Part model, mm, in its own coordinate system. A direction names the side the tool comes from. Round coordinates to 2 decimals unless told otherwise and drop trailing zeros. Loops run counter-clockwise (first coordinate to the right, second up) from the corner with the lowest first, then second, coordinate; pieces in that order, holes last.
from build123d import *

# Parameters (mm, degrees)
SKETCH1_R           = 1.7
BOSS_EXTRUDE1_DEPTH = 70
SKETCH2_W           = 60
SKETCH2_H           = 10
CUT_EXTRUDE1_DEPTH  = 25
BOSS_EXTRUDE2_DEPTH = 5
SKETCH4_W           = 10
SKETCH4_H           = 60
CUT_EXTRUDE2_DEPTH  = 20
BOSS_EXTRUDE3_DEPTH = 5


with BuildPart() as part:
    # Sketch1 → Boss-Extrude1 (new body)
    with BuildSketch(Plane.XY.offset(246.476360497)):
        Polygon((-42.55341426, 305.4352577), (-42.55341426, 275.4352577), (-22.55341426, 275.4352577), (-22.55341426, 285.4352577), (-12.649269186, 285.4352577), (-12.649269186, 305.4352577), align=None)
        with Locations((-17.55341426, 295.4352577)):
            Circle(SKETCH1_R, mode=Mode.SUBTRACT)
        with Locations((-32.55341426, 280.4352577)):
            Circle(SKETCH1_R, mode=Mode.SUBTRACT)
    extrude(amount=BOSS_EXTRUDE1_DEPTH)

    # Sketch2 → Cut-Extrude1 (cut)
    with BuildSketch(Plane.ZY.offset(42.55341426)):
        with Locations((281.476360497, 280.4352577)):
            Rectangle(SKETCH2_W, SKETCH2_H)
    extrude(amount=-CUT_EXTRUDE1_DEPTH, mode=Mode.SUBTRACT)

    # Sketch3 → Boss-Extrude2 (add)
    with BuildSketch(Plane.ZY.offset(42.55341426)):
        Polygon((311.476360497, 275.4352577), (301.476360497, 285.4352577), (261.476360497, 285.4352577), (251.476360497, 275.4352577), (246.476360497, 275.4352577), (246.476360497, 305.4352577), (316.476360497, 305.4352577), (316.476360497, 275.4352577), align=None)
    extrude(amount=-BOSS_EXTRUDE2_DEPTH)

    # Sketch4 → Cut-Extrude2 (cut)
    with BuildSketch(Plane(origin=(0, 305.4352577, 0), x_dir=(1, 0, 0), z_dir=(0, 1, 0))):
        with Locations((-17.649269186, -281.476360497)):
            Rectangle(SKETCH4_W, SKETCH4_H)
    extrude(amount=-CUT_EXTRUDE2_DEPTH, mode=Mode.SUBTRACT)

    # Sketch5 → Boss-Extrude3 (add)
    with BuildSketch(Plane(origin=(0, 305.4352577, 0), x_dir=(1, 0, 0), z_dir=(0, 1, 0))):
        Polygon((-12.649269186, -311.476360497), (-22.649269186, -301.476360497), (-22.649269186, -261.476360497), (-12.649269186, -251.476360497), (-12.649269186, -246.476360497), (-42.55341426, -246.476360497), (-42.55341426, -316.476360497), (-12.649269186, -316.476360497), align=None)
    extrude(amount=-BOSS_EXTRUDE3_DEPTH)


solid = part.part
1) Slice it at B-B, the plane x = -24.5. Give the cut face in (y, z).
Values:
outline: (275.44, 246.48) - (305.44, 246.48) - (305.44, 316.48) - (275.44, 316.48) - (275.44, 311.48) - (285.44, 311.48) - (285.44, 251.48) - (275.44, 251.48) - close
2) Wall check: line 1 along Z through (x, y) = (-15.25, 294.75); line 2 along Y through (x, z) = (-16, 254); line 3 along X through (y, z) = (289, 294). Give the ranges that are in metal, low to high.
Values:
line 1: z = 246.48 to 251.48, 311.48 to 316.48
line 2: y = 300.44 to 305.44
line 3: x = -42.55 to -22.65
3) Drop flat-ended pins along their axis: pin 1 Ø2.5 at (x, z) = (-15.5, 313.5) entering from -Y; pin 2 Ø16 at (y, z) = (296.5, 292) entering from +X; pin 3 Ø3 at (x, y) = (-32.55, 280.44) entering from +Z; pin 4 Ø8 at (y, z) = (279, 256) entering from +X. Give the stop position or say it passes through.
Values:
pin 1: stops at y = 285.44
pin 2: stops at x = -22.65
pin 3: passes through
pin 4: stops at x = -37.55
4) Tool access for faces 1 (the face through (-20, 300.435, 309)), 2 (the face through (-17.579, 302.97, 306.546)), 3 (the face through (-22.553, 280, 249)), 4 (the face through (-40.088, 280.365, 306.546)): list every direction of +Z, -Z, +X, -X, +Y, -Y with a clear straight run to the whole face (end or side of a thin tool).
Values:
face 1: +X, -Y
face 2: +X, +Y, -Y
face 3: +Z, -Z, +X, -Y
face 4: +X, -X, -Y
5) Slice it at A-A, the plane y = 301.5. Give the cut face in (x, z), then the cut area to 3 significant figures.
Values:
outline: (-42.55, 246.48) - (-12.65, 246.48) - (-12.65, 251.48) - (-22.65, 261.48) - (-22.65, 301.48) - (-12.65, 311.48) - (-12.65, 316.48) - (-42.55, 316.48) - close
area: 1,590 mm2
6) Slice it at D-D, the plane z = 268. Give the cut face in (x, y), then the cut area to 3 significant figures.
Values:
outline: (-42.55, 285.44) - (-22.65, 285.44) - (-22.65, 305.44) - (-42.55, 305.44) - close
area: 398 mm2
7) Slice it at C-C, the plane y = 278. Give the cut face in (x, z), then the cut area to 3 significant figures.
Values:
outline: (-42.55, 246.48) - (-22.55, 246.48) - (-22.55, 251.48) - (-37.55, 251.48) - (-37.55, 254.04) - (-42.55, 254.04) - close; (-42.55, 308.91) - (-37.55, 308.91) - (-37.55, 311.48) - (-22.55, 311.48) - (-22.55, 316.48) - (-42.55, 316.48) - close
area: 226 mm2
8) Mould opens along Y. For faces 5 (the face through (-25, 285, 311.476)), 6 (the face through (-18, 285.435, 314)), 7 (the face through (-17.77, 297.12, 248.94)) say: released by +Y, released by -Y, zero draft, split by the parting line, or undercut.
Values:
face 5: zero draft
face 6: released by -Y
face 7: undercut
